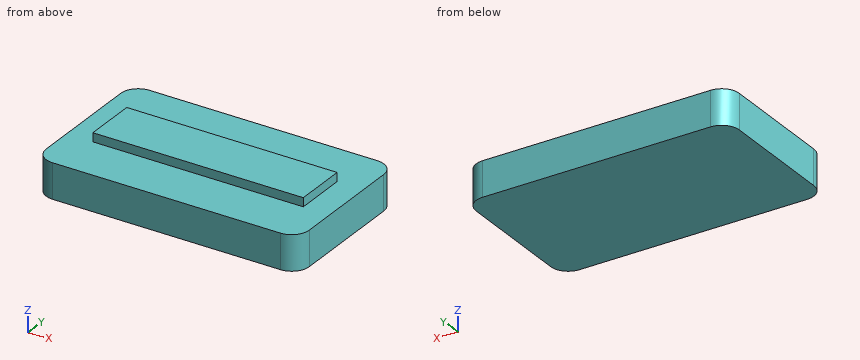
Solid Edge part; units mm, degrees
sketch "Sketch1" plane through (0, 0, 0) normal (0, 0, 1) x (1, 0, 0)
  line L0 (-75, -43) -> (75, -43)
  line L1 (75, -43) -> (75, 43)
  line L2 (75, 43) -> (-75, 43)
  line L3 (-75, 43) -> (-75, -43)
extrude "Protrusion1" add sketch "Sketch1" against normal blind 20
sketch "Sketch2" plane through (0, 0, 0) normal (0, 0, 1) x (1, 0, 0)
  line L0 (-60, -15) -> (60, -15)
  line L1 (60, -15) -> (60, 15)
  line L2 (60, 15) -> (-60, 15)
  line L3 (-60, 15) -> (-60, -15)
extrude "ExtrudedProtrusion_2" add sketch "Sketch2" along normal blind 5
fillet "Round_1" radius 10 4 edges at (75, -43, -10) (75, 43, -10) (-75, -43, -10) (-75, 43, -10)
Work out the finished part from the listing and answer in its coordinate system (mm). Round coordinates to 2 decimals unless told otherwise and drop trailing zeros. Loops run counter-clockwise (first coordinate to the right, second up) from the corner with the lowest first, then second, coordinate; pieces in that order, holes last. Notation, with made-up numbers: (24, 84.5) -> (39, 84.5) arc R21 cw to (39, 107.5) -> close; hole circle Ø9 at (46, 24.5). An arc over 180 degrees is marked (long way). Write each question's results on one line, items separated by ' | '. Start each with the question number.
1. Section A-A (y = 7) is taken. Determine the outline of the cut face in (x, z), plus the area to 3 significant figures.
2. Section C-C (x = 63.5) is taken. Determine the outline of the cut face in (y, z).
3. Section B-B (x = 43.5) is taken. Determine the outline of the cut face in (y, z).
4. Section D-D (y = 29) is taken. Determine the outline of the cut face in (x, z).
5. Find the intervals of material crossed by probe 1 along Z at (x, y) = (19, 31.5); probe 2 along Y at (x, z) = (-6.5, 4); probe 3 along X at (y, z) = (34, -14.25), in increasing order. Write a range as from..to.
6. Given pin 1 Ø2.5 at (y, z) = (-6, 2.5) entering from +X; pin 2 Ø2.5 at (y, z) = (-4, 3.5) entering from -X; pin 3 Ø2.5 at (x, z) = (5.5, 3) entering from -Y, each flat-ended and moving along its own axis, determine where each tip first touches the part or whether it passes through.
Evaluation:
1) outline: (-75, -20) -> (75, -20) -> (75, 0) -> (60, 0) -> (60, 5) -> (-60, 5) -> (-60, 0) -> (-75, 0) -> close | area: 3,600 mm2
2) outline: (-43, -20) -> (43, -20) -> (43, 0) -> (-43, 0) -> close
3) outline: (-43, -20) -> (43, -20) -> (43, 0) -> (15, 0) -> (15, 5) -> (-15, 5) -> (-15, 0) -> (-43, 0) -> close
4) outline: (-75, -20) -> (75, -20) -> (75, 0) -> (-75, 0) -> close
5) probe 1: z = -20..0 | probe 2: y = -15..15 | probe 3: x = -74.95..74.95
6) pin 1: stops at x = 60 | pin 2: stops at x = -60 | pin 3: stops at y = -15
